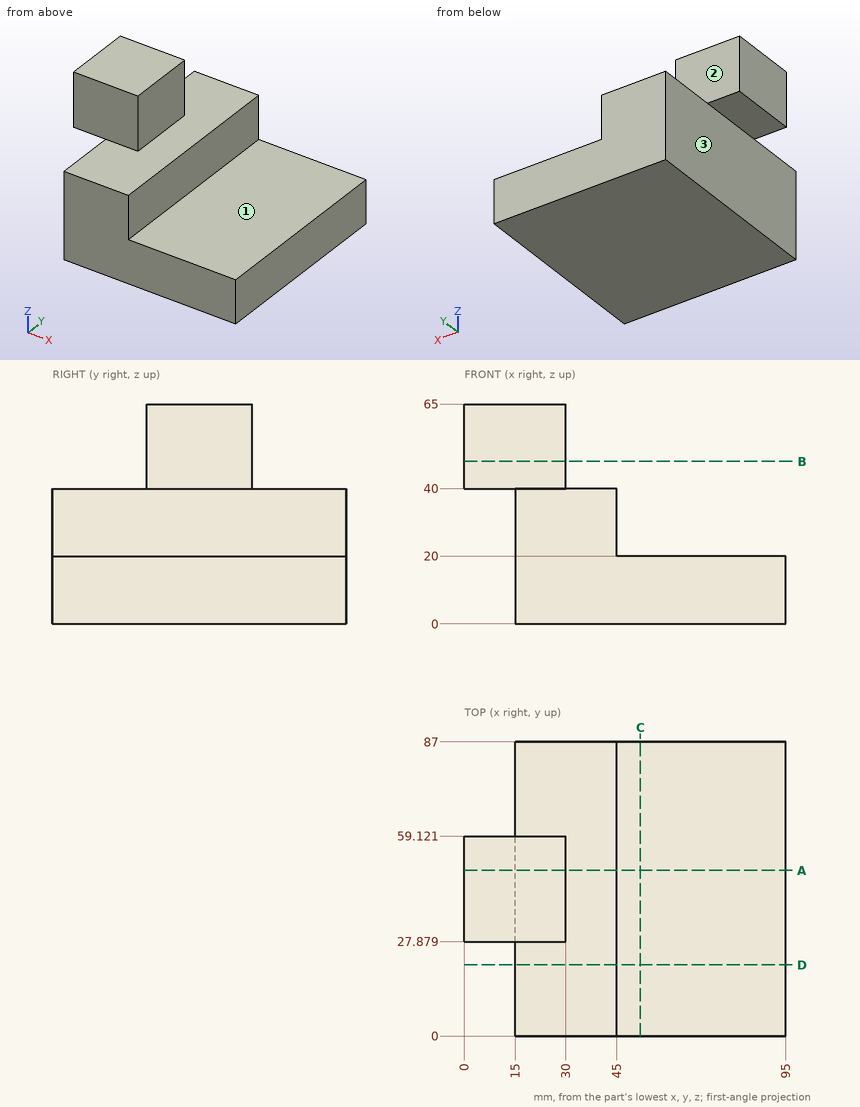
Part print with two shaded views. Sizes in mm from the minimum x, y, z corner. A direction names the side the tool comes from. Round coordinates to 2 decimals unless told otherwise and drop trailing zeros. Loops run counter-clockwise (first coordinate to the right, second up) from the corner with the lowest first, then second, coordinate; pieces in that order, holes last.
Item 1: Saw through at C-C (x = 52). List the corners of the cut face in (y, z).
Item 2: Pin check, flat tips, straight feed: P1, Ø16.5, axis at x = 6, y = 46, coming from the -Z side; P2, Ø10, axis at x = 81, y = 14, coming from the +Z side; P3, Ø10, axis at y = 16.5, z = 37.5, coming from the -X side. Stop position of each tip, or through.
Item 3: Saw through at D-D (y = 21). List the corners of the cut face in (x, z), then the cut area to 3 significant figures.
Item 4: Drill centre lines: line 1 along Y through (x, z) = (11, 58); line 2 along Z through (x, y) = (7, 54); line 3 along X through (y, z) = (44.5, 53). Where is each one in solid material? Low to high.
Item 5: Saw through at B-B (z = 48). List the corners of the cut face in (x, y), then the cut area to 3 significant figures.
Item 6: Which spindle directions (+Z, -Z, +X, -X, +Y, -Y) get a long thin tool onto all of the face, cutting with end or side? Do the marked faces 1, 2 and 3. Say none if no direction does.
Item 7: Saw through at A-A (y = 49). List the corners of the cut face in (x, z), then the cut area to 3 significant figures.
Worked answers:
1. outline: (0, 0) - (87, 0) - (87, 20) - (0, 20) - close
2. P1: stops at z = 40
2. P2: stops at z = 20
2. P3: stops at x = 15
3. outline: (15, 0) - (95, 0) - (95, 20) - (45, 20) - (45, 40) - (15, 40) - close
3. area: 2,200 mm2
4. line 1: y = 27.88 to 59.12
4. line 2: z = 40 to 65
4. line 3: x = 0 to 30
5. outline: (0, 27.88) - (30, 27.88) - (30, 59.12) - (0, 59.12) - close
5. area: 937 mm2
6. face 1: +Z, +X, +Y, -Y
6. face 2: +Z, +X, -X, +Y
6. face 3: -Z, -X, +Y, -Y
7. outline: (0, 40) - (15, 40) - (15, 0) - (95, 0) - (95, 20) - (45, 20) - (45, 40) - (30, 40) - (30, 65) - (0, 65) - close
7. area: 2,950 mm2
